Design review of the part built by this model. Coordinates are the model's own, in mm. A direction names the side the tool comes from. Coordinates: 2 decimals unless noted, no trailing zeros. Loops run counter-clockwise (first coordinate to the right, second up) from the corner with the lowest first, then second, coordinate; pieces in that order, holes last.
from build123d import *

# Parameters (mm, degrees)
F0_W      = 2.65
F0_H      = 12.7
F0_W_2    = 6.1
F0_H_2    = 3.45
F1_DEPTH  = 0.4
F2_W      = 2.4
F2_H      = 1.035
F3_DEPTH  = 1
F4_W      = 8.2
F4_H      = 6.3
F5_DEPTH  = 0.2
F6_W      = 8.2
F6_H      = 3.8
F7_DEPTH  = 5.3
F8_W      = 11.4
F8_H      = 12.7
F9_DEPTH  = 7.2
F10_W     = 1
F10_H     = 3
F11_DEPTH = 0.5
F12_W     = 2.8
F12_H     = 0.8
F13_DEPTH = 4.5
F14_R     = 1
F15_SIZE  = 0.5
F16_W     = 0.8
F16_H     = 11.5
F17_DEPTH = 1.5
F18_R     = 0.2
F19_W     = 0.2
F19_H     = 0.2
F20_DEPTH = 25


with BuildPart() as f1:
    # F0 (on Top) → F1 (new body)
    with BuildSketch(Plane.XY):
        with Locations((4.375, 0)):
            Rectangle(F0_W, F0_H)
        with Locations((0, -8.075)):
            Rectangle(F0_W_2, F0_H_2)
        Rectangle(F0_W_2, F0_H)
        with Locations((-4.375, 0)):
            Rectangle(F0_W, F0_H)
        with Locations((0, 8.075)):
            Rectangle(F0_W_2, F0_H_2)
    extrude(amount=F1_DEPTH)

    # F2 (on face) → F3 (cut)
    with BuildSketch(Plane.XY.offset(0.4)):
        with BuildLine():
            ThreePointArc((-1.2, 8.765), (0, 7.565), (1.2, 8.765))
            Line((1.2, 8.765), (-1.2, 8.765))
        make_face()
        with Locations((0, 9.2825)):
            Rectangle(F2_W, F2_H)
        with BuildLine():
            Line((-1.2, -8.765), (1.2, -8.765))
            ThreePointArc((1.2, -8.765), (0, -7.565), (-1.2, -8.765))
        make_face()
        with Locations((0, -9.2825)):
            Rectangle(F2_W, F2_H)
    extrude(amount=-F3_DEPTH, mode=Mode.SUBTRACT)

    # F4 (on face) → F5 (cut)
    with BuildSketch(Plane.XY.offset(0.4)):
        Rectangle(F4_W, F4_H)
    extrude(amount=-F5_DEPTH, mode=Mode.SUBTRACT)

    # F6 (on face) → F7 (join)
    with BuildSketch(Plane.XY.offset(0.2)):
        Rectangle(F6_W, F6_H)
    extrude(amount=F7_DEPTH)

    # F8 (on face) → F9 (join)
    with BuildSketch(Plane(origin=(0, 0, 0), x_dir=(1, 0, 0), z_dir=(0, 0, -1))):
        Rectangle(F8_W, F8_H)
    extrude(amount=F9_DEPTH)

    # F10 (on face) → F11 (join)
    with BuildSketch(Plane.YZ.offset(5.7)):
        with Locations((4.5, -5.7)):
            Rectangle(F10_W, F10_H)
        with Locations((-4.5, -5.7)):
            Rectangle(F10_W, F10_H)
    extrude(amount=F11_DEPTH)

    # F12 (on face) → F13 (join)
    with BuildSketch(Plane(origin=(0, 0, -7.2), x_dir=(1, 0, 0), z_dir=(0, 0, -1))):
        with Locations((2.4, -4.7)):
            Rectangle(F12_W, F12_H)
        with Locations((2.4, 0)):
            Rectangle(F12_W, F12_H)
        with Locations((2.4, 4.7)):
            Rectangle(F12_W, F12_H)
        with Locations((-2.4, -4.7)):
            Rectangle(F12_W, F12_H)
        with Locations((-2.4, 0)):
            Rectangle(F12_W, F12_H)
        with Locations((-2.4, 4.7)):
            Rectangle(F12_W, F12_H)
    extrude(amount=F13_DEPTH)

    # F14
    f14_edges = [f1.edges().sort_by_distance(p)[0] for p in [
        (3.05, 6.35, 0.2),
        (-3.05, 6.35, 0.2),
        (3.05, -6.35, 0.2),
        (-3.05, -6.35, 0.2),
    ]]
    fillet(f14_edges, radius=F14_R)

    # F15
    f15_edges = [f1.edges().sort_by_distance(p)[0] for p in [
        (1, 4.7, -11.7),
        (3.8, 4.7, -11.7),
        (-1, 4.7, -11.7),
        (-3.8, 4.7, -11.7),
        (1, 0, -11.7),
        (3.8, 0, -11.7),
        (-1, 0, -11.7),
        (-3.8, 0, -11.7),
        (-3.8, -4.7, -11.7),
        (-1, -4.7, -11.7),
        (1, -4.7, -11.7),
        (3.8, -4.7, -11.7),
    ]]
    chamfer(f15_edges, length=F15_SIZE)

    # F16 (on face) → F17 (join)
    with BuildSketch(Plane(origin=(0, 0, -7.2), x_dir=(1, 0, 0), z_dir=(0, 0, -1))):
        Rectangle(F16_W, F16_H)
    extrude(amount=F17_DEPTH)

    # F18
    f18_edges = [f1.edges().sort_by_distance(p)[0] for p in [
        (0, -5.75, -8.7),
        (0, 5.75, -8.7),
        (0.4, 0, -8.7),
        (-0.4, 0, -8.7),
        (6.2, -5, -5.7),
        (6.2, -4, -5.7),
        (6.2, 5, -5.7),
        (6.2, 4, -5.7),
    ]]
    fillet(f18_edges, radius=F18_R)

    # F19 (on face) → F20 (cut)
    with BuildSketch(Plane.YZ.offset(4.1)):
        with Locations((-1.4904041938, 5.4)):
            Rectangle(F19_W, F19_H)
        with Locations((-1.1904041938, 5.4)):
            Rectangle(F19_W, F19_H)
        with Locations((-0.8904041938, 5.4)):
            Rectangle(F19_W, F19_H)
        with Locations((-0.5904041938, 5.4)):
            Rectangle(F19_W, F19_H)
        with Locations((-0.2904041938, 5.4)):
            Rectangle(F19_W, F19_H)
        with Locations((0.0095958062, 5.4)):
            Rectangle(F19_W, F19_H)
        with Locations((0.3095958062, 5.4)):
            Rectangle(F19_W, F19_H)
        with Locations((0.6095958062, 5.4)):
            Rectangle(F19_W, F19_H)
        with Locations((0.9095958062, 5.4)):
            Rectangle(F19_W, F19_H)
        with Locations((1.2095958062, 5.4)):
            Rectangle(F19_W, F19_H)
        with Locations((1.5095958062, 5.4)):
            Rectangle(F19_W, F19_H)
    extrude(amount=-F20_DEPTH, mode=Mode.SUBTRACT)


solid = f1.part
Q1. Take a section at A-A, the plane z = -10.25. Write out the cut boundary in (x, y), then the cut area to 3 significant figures.
Q2. Take a section at C-C, the plane z = 1.75. Write out the cut boundary in (x, y), then the cut area to 3 significant figures.
Q3. Machinability: for faces 5 (the flat face through (1, 4.7, -9.2)), 6 (the flat face through (-2, -0.4, -9)), 7 (the flat face through (-2, 5.1, -9)), 8 (the flat face through (-3.8, 4.7, -9.2)), which of the approach directions +Z, -Z, +X, -X, +Y, -Y give a long, thin tool a straight path to every point of the face, cutting with its end or side? Answer none if there is none.
Q4. Take a section at B-B, the plane x = 5.25. Write out the cut boundary in (y, z).
Q5. Clearance check with flat-ended pins moving along their axes: pin 1 Ø0.6 at (y, z) = (-5, -9.5) entering from +X; pin 2 Ø0.8 at (x, z) = (2, -9.5) entering from -Y; pin 3 Ø1 at (x, z) = (0, -10) entering from +Y; pin 4 Ø1 at (x, z) = (-1, -9) entering from +Y. State where each tip first meets the part, or that it passes through.
Q6. The part is to be moulded in two halves that separate along X. For faces 1 (the cylindrical face through (3.351, -6.635, 0.203)), 2 (the flat face through (0, 6.35, -3)), 3 (the flat face through (-0.1, -2.5, 0.2)), 4 (the flat face through (-0.1, 2.5, 0.2)), say which applies: pulls with the +X half, pulls with the -X half, needs draft (parallel to the pull), parting line crosses it, or undercut.
Q7. For line 1 (Y direction, x = 2.75, z = -0.25); line 2 (Z direction, x = 5, y = 2.5); line 3 (Z direction, x = 0.75, y = 7.5), list the stretches that pass through material, from the lowest coordinate up.
Entries:
1. outline: (-3.8, -5.1) - (-1, -5.1) - (-1, -4.3) - (-3.8, -4.3) - close; (-3.8, -0.4) - (-1, -0.4) - (-1, 0.4) - (-3.8, 0.4) - close; (-3.8, 4.3) - (-1, 4.3) - (-1, 5.1) - (-3.8, 5.1) - close; (1, -5.1) - (3.8, -5.1) - (3.8, -4.3) - (1, -4.3) - close; (1, -0.4) - (3.8, -0.4) - (3.8, 0.4) - (1, 0.4) - close; (1, 4.3) - (3.8, 4.3) - (3.8, 5.1) - (1, 5.1) - close
1. area: 13.4 mm2
2. outline: (-4.1, -1.9) - (4.1, -1.9) - (4.1, 1.9) - (-4.1, 1.9) - close
2. area: 31.2 mm2
3. face 5: -Z, +Y, -Y
3. face 6: -Z, -X
3. face 7: -Z, -X, +Y
3. face 8: -Z, -X, +Y, -Y
4. outline: (-6.35, -7.2) - (6.35, -7.2) - (6.35, 0.4) - (-6.35, 0.4) - close
5. pin 1: stops at x = 3.8
5. pin 2: stops at y = -5.1
5. pin 3: passes through
5. pin 4: stops at y = 5.1
6. face 1: pulls with the +X half
6. face 2: needs draft
6. face 3: undercut
6. face 4: undercut
7. line 1: y = -6.35 to 6.35
7. line 2: z = -7.2 to 0.4
7. line 3: z = 0 to 0.4
